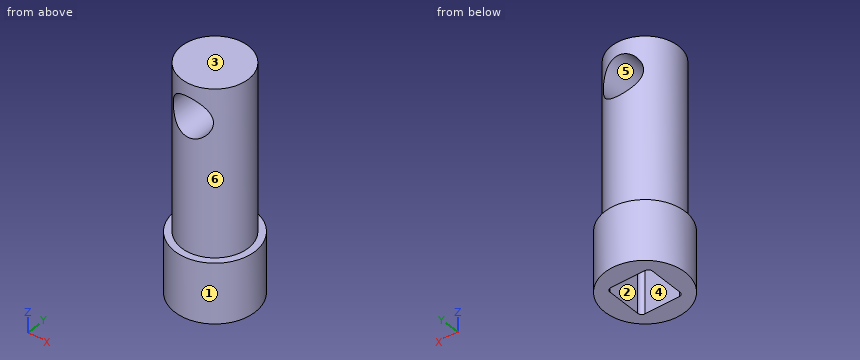
from build123d import *

# Parameters (mm, degrees)
SKETCH_1_R          = 5
EXTRUDE_1_DEPTH     = 34
SKETCH_4_R          = 6
EXTRUDE_2_DEPTH     = 9
CUT_EXTRUDE_1_DEPTH = 8
SKETCH_3_R          = 3
CUT_EXTRUDE_2_DEPTH = 12


with BuildPart() as part:
    # 草图1 → 凸台-拉伸1 (new body)
    with BuildSketch(Plane.XY):
        Circle(SKETCH_1_R)
    extrude(amount=EXTRUDE_1_DEPTH)

    # 草图4 → 凸台-拉伸2 (add)
    with BuildSketch(Plane.XY):
        Circle(SKETCH_4_R)
    extrude(amount=EXTRUDE_2_DEPTH)

    # 草图2 → 切除-拉伸1 (cut)
    with BuildSketch(Plane(origin=(0, 0, 0), x_dir=(-1, 0, 0), z_dir=(0, 0, -1))):
        with BuildLine():
            Line((2.565, -3.165), (-2.565, -3.165))
            ThreePointArc((-2.565, -3.165), (-2.989264069, -2.989264069), (-3.165, -2.565))
            Line((-3.165, -2.565), (-3.165, 2.565))
            ThreePointArc((-3.165, 2.565), (-2.989264069, 2.989264069), (-2.565, 3.165))
            Line((-2.565, 3.165), (2.565, 3.165))
            ThreePointArc((2.565, 3.165), (2.989264069, 2.989264069), (3.165, 2.565))
            Line((3.165, 2.565), (3.165, -2.565))
            ThreePointArc((3.165, -2.565), (2.989264069, -2.989264069), (2.565, -3.165))
        make_face()
    extrude(amount=-CUT_EXTRUDE_1_DEPTH, mode=Mode.SUBTRACT)

    # 草图3 → 切除-拉伸2 (cut, through all)
    with BuildSketch(Plane(origin=(0, -5, 0), x_dir=(-1, 0, 0), z_dir=(0, -1, 0))):
        with Locations((0, -29)):
            Circle(SKETCH_3_R)
    extrude(amount=-CUT_EXTRUDE_2_DEPTH, mode=Mode.SUBTRACT)


solid = part.part
The listing builds one solid part. Answer for the finished solid, in the listing's coordinates (mm). Face numbers are marked on the shaded views. A direction names the side the tool comes from. Round coordinates to 2 decimals unless told otherwise and drop trailing zeros. Write each loop counter-clockwise with the first axis right and the second up, starting at its lowest first coordinate (ties: lowest second). Pieces come first, ordered by that corner, then holes. Notation, with made-up numbers: (73.5, -39.75) - (98.5, -39.75) arc R26 cw to (98.5, -8.75) - close; hole circle Ø11 at (86.5, 10.5). An arc over 180 degrees is marked (long way). Use one line per item in the form item = value. Start each with the question number.
Item 1: A cutting plane is placed at D-D (z = 6.5). Write down the section's boundary in (x, y) (3 decimals).
Item 2: A tool of negligible diameter and unlimited length cuts with its end or side. For the marked faces 4, 5 and 6, from which of +Z, -Z, +X, -X, +Y, -Y can it reach the whole face along a straight path? Write none if from no direction.
Item 3: A cutting plane is placed at B-B (x = 0). Write down the section's boundary in (y, z) (3 decimals).
Item 4: A cutting plane is placed at A-A (y = 0). Write down the section's boundary in (x, z) (3 decimals).
Item 5: Flat-ended cylindrical pins translate along their axes: pin 1 Ø2 at (y, z) = (1, 28.5) entering from +X; pin 2 Ø2 at (x, z) = (-4, 16.5) entering from -Y; pin 3 Ø1.5 at (x, z) = (1, 4.5) entering from +Y. Find the tip coordinate at first contact, or state that the pin passes through.
Item 6: Find the intervals of material crossed by line 1 (Z direction, x = 0, y = 2.5); line 2 (X direction, y = -1, z = 29); line 3 (Z direction, x = -1, y = -2.75), in increasing order. Write a range as [from, to].
Item 7: Determine the mould class of the marked faces 1, 2 and 3 for opening direction Y: +Y half, -Y half, draft (parallel to the pull), parting line (faces both ways), or undercut.
Item 8: A cutting plane is placed at C-C (z = 29). Write down the section's boundary in (x, y).
The answers:
q1.outline = circle Ø12 at (0, 0); hole (-3.165, -2.565) arc R0.6 ccw to (-2.565, -3.165) - (2.565, -3.165) arc R0.6 ccw to (3.165, -2.565) - (3.165, 2.565) arc R0.6 ccw to (2.565, 3.165) - (-2.565, 3.165) arc R0.6 ccw to (-3.165, 2.565) - close
q2.face_4 = -Z
q2.face_5 = +Y, -Y
q2.face_6 = +Z
q3.outline = (-6, 0) - (-3.165, 0) - (-3.165, 8) - (3.165, 8) - (3.165, 0) - (6, 0) - (6, 9) - (5, 9) - (5, 26) - (-5, 26) - (-5, 9) - (-6, 9) - close; (-5, 32) - (5, 32) - (5, 34) - (-5, 34) - close
q4.outline = (-6, 0) - (-3.165, 0) - (-3.165, 8) - (3.165, 8) - (3.165, 0) - (6, 0) - (6, 9) - (5, 9) - (5, 34) - (-5, 34) - (-5, 9) - (-6, 9) - close; hole circle Ø6 at (0, 29)
q5.pin_1 = 5
q5.pin_2 = -4
q5.pin_3 = 5.99
q6.line_1 = [8, 26], [32, 34]
q6.line_2 = [-4.9, -3], [3, 4.9]
q6.line_3 = [8, 26.17], [31.83, 34]
q7.face_1 = parting line
q7.face_2 = undercut
q7.face_3 = draft
q8.outline = (-3, -4) - (-3, 4) arc R5 ccw to start; (3, -4) arc R5 ccw to (3, 4) - close
